```python
from build123d import *

# Parameters (mm, degrees)
SKETCH1_W                   = 200
SKETCH1_H                   = 200
BOSS_EXTRUDE1_DEPTH         = 10
CUT_EXTRUDE2_DEPTH          = 284.019433962
CUT_EXTRUDE2_DEPTH_BACK     = 284.019433962
SKETCH2_R                   = 13
TAP_DRILL_FOR_M3X0_5_TAP1_D = 2.6


with BuildPart() as part:
    # Sketch1 → Boss-Extrude1 (new body)
    with BuildSketch(Plane(origin=(0, 0, 0), x_dir=(1, 0, 0), z_dir=(0, 1, 0))):
        with Locations((100, 100)):
            Rectangle(SKETCH1_W, SKETCH1_H)
    extrude(amount=BOSS_EXTRUDE1_DEPTH)

    # Sketch2 → Cut-Extrude2 (cut, two sides: drawn at the far end of the back side and taken through both)
    with BuildSketch(Plane(origin=(0, 0, 0), x_dir=(1, 0, 0), z_dir=(0, 1, 0)).offset(-CUT_EXTRUDE2_DEPTH_BACK)):
        with Locations(Location((100, 100, 0), (0, 0, 270))):
            Circle(SKETCH2_R)
    extrude(amount=CUT_EXTRUDE2_DEPTH + CUT_EXTRUDE2_DEPTH_BACK, mode=Mode.SUBTRACT)

    # Tap Drill for M3x0.5 Tap1 (through all)
    with Locations(Plane(origin=(0, 10, 0), x_dir=(1, 0, 0), z_dir=(0, 1, 0))):
        with Locations((20, 180), (180, 180), (180, 20), (20, 20), (100, 117), (117, 100), (100, 83), (83, 100)):
            Hole(TAP_DRILL_FOR_M3X0_5_TAP1_D / 2)


solid = part.part
```
CAD build for the part. Positions are in the model's coordinates, mm. Round coordinates to 2 decimals unless told otherwise and drop trailing zeros. Loops run counter-clockwise (first coordinate to the right, second up) from the corner with the lowest first, then second, coordinate; pieces in that order, holes last. Notation, with made-up numbers: M 4,46.25 L 46,46.25 A21 ccw 46,71.25 Z; hole C -11.75,-3 d6. An arc over 180 degrees is marked long. Return JSON: item names as keys, results as strings. Group by question number.
(1) Drop flat-ended pins along their axis: P1, Ø5, axis at x = 54.5, y = 3.5, coming from the +Z side; P2, Ø2.5, axis at x = 20, z = -20, coming from the +Y side. Give the stop position or say it passes through.
(2) Saw through at B-B, the plane z = -91.5. List the corners of the cut face in (x, y).
(3) Mould opens along Z. For faces 1 (the cylindrical face through (92.09, 4.93, -110.316)), 2 (the flat face through (99, 5, 0)), 3 (the flat face through (76, 0, -101)) say: +Z half, -Z half, draft (parallel to the pull), parting line (faces both ways), or undercut.
(4) Wall check: probe 1 along Z at (x, y) = (20, 7.5); probe 2 along Z at (x, y) = (100, 7.5); probe 3 along X at (y, z) = (5.75, -180). Give the ranges that are in metal, low to high. Write a range as [from, to].
(5) Saw through at A-A, the plane x = 106. List the corners of the cut face in (y, z).
Answer list:
{
 "1": {"P1": "z = 0", "P2": "through"},
 "2": {"outline": "M 0,0 L 90.16,0 L 90.16,10 L 0,10 Z; M 109.84,0 L 200,0 L 200,10 L 109.84,10 Z"},
 "3": {"face 1": "undercut", "face 2": "+Z half", "face 3": "draft"},
 "4": {"probe 1": "[-200, -181.3], [-178.7, -21.3], [-18.7, 0]", "probe 2": "[-200, -118.3], [-115.7, -113], [-87, -84.3], [-81.7, 0]", "probe 3": "[0, 18.7], [21.3, 178.7], [181.3, 200]"},
 "5": {"outline": "M 0,-200 L 10,-200 L 10,-111.53 L 0,-111.53 Z; M 0,-88.47 L 10,-88.47 L 10,0 L 0,0 Z"}
}
